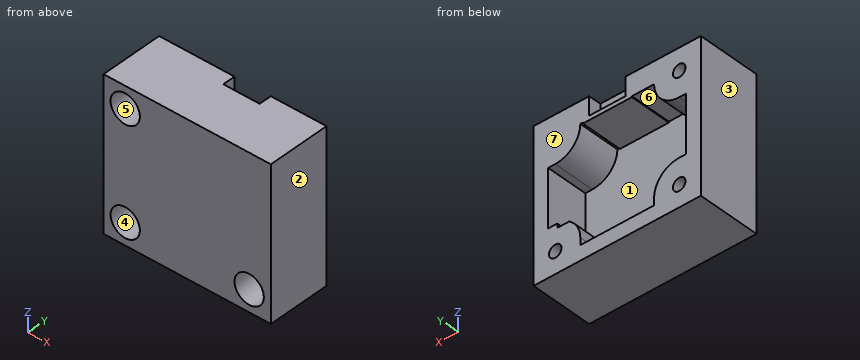
Autodesk Inventor part; units mm, degrees
ref_plane "YZ Plane" through (0, 0, 0) normal (1, 0, 0) x (0, 1, 0)
ref_plane "XZ Plane" through (0, 0, 0) normal (0, 1, 0) x (-1, 0, 0)
ref_plane "XY Plane" through (0, 0, 0) normal (0, 0, 1) x (1, 0, 0)
sketch "Эскиз1" plane through (0, 0, 0) normal (0, 1, 0) x (-1, 0, 0)
  line L0 (18, -16) -> (-18, -16)
  line L1 (-18, -16) -> (-18, 16)
  line L2 (-18, 16) -> (18, 16)
  line L3 (18, 16) -> (18, -16)
  line L4 (0, -25.2) -> (0, 25.2)
  line L5 (28, 0) -> (-28, 0)
  line L6 (14.82, -12.82) -> (-14.82, -12.82)
  line L7 (-14.82, -12.82) -> (-14.82, 12.82)
  line L8 (-14.82, 12.82) -> (14.82, 12.82)
  line L9 (14.82, 12.82) -> (14.82, -12.82)
  circle A0 centre (14.82, -12.82) radius 1.5
  circle A1 centre (14.82, 12.82) radius 1.5
  circle A2 centre (-14.82, 12.82) radius 1.5
  circle A3 centre (-14.82, -12.82) radius 1.5
  arc A4 (14.82, -6.82) -> (8.82, -12.82) centre (14.82, -12.82) ccw
  arc A5 (-8.82, -12.82) -> (-14.82, -6.82) centre (-14.82, -12.82) ccw
  arc A6 (8.82, 12.82) -> (14.82, 6.82) centre (14.82, 12.82) ccw
  arc A7 (-14.82, 6.82) -> (-8.82, 12.82) centre (-14.82, 12.82) ccw
  line L10 (20, -18) -> (-20, -18)
  line L11 (-20, -18) -> (-20, 18)
  line L12 (-20, 18) -> (20, 18)
  line L13 (20, 18) -> (20, -18)
  line L14 (-8.82, -12.82) -> (-8.82, -16)
  line L15 (8.82, -12.82) -> (8.82, -16)
  line L16 (14.82, -6.82) -> (18, -6.82)
  line L17 (14.82, 6.82) -> (18, 6.82)
  line L18 (8.82, 12.82) -> (8.82, 16)
  line L19 (-14.82, -6.82) -> (-20, -6.82)
  line L20 (-14.82, 6.82) -> (-20, 6.82)
  line L21 (-8.82, 12.82) -> (-8.82, 18)
  line L22 (-18, -6.82) -> (-18, 6.82)
  line L23 (8.82, 16) -> (-8.82, 16)
  line L24 (2, 13.6) -> (-6.7, 13.6)
  line L25 (-6.7, 13.6) -> (-6.7, 18)
  line L26 (3.5, 16) -> (3.5, 12.6)
  line L27 (3.5, 12.6) -> (-8.2, 12.6)
  line L28 (-8.2, 12.6) -> (-8.2, 16)
  line L29 (2, 13.6) -> (2, 18)
  circle A8 centre (-14.82, -12.82) radius 3.5
  circle A9 centre (14.82, -12.82) radius 3.5
  circle A10 centre (14.82, 12.82) radius 3.5
  circle A11 centre (-14.82, 12.82) radius 4
  line L30 (18, 6.82) -> (16.5, 6.82)
  line L31 (16.5, 6.82) -> (16.5, -6.82)
  line L32 (16.5, -6.82) -> (18, -6.82)
  line L33 (18, -6.82) -> (18, 6.82)
  line L34 (8.82, 16) -> (3.5, 16)
  line L35 (3.5, 16) -> (3.5, 14.5)
  line L36 (3.5, 14.5) -> (8.82, 14.5)
  line L37 (8.82, 14.5) -> (8.82, 16)
  line L38 (-8.2, 16) -> (-8.82, 16)
  line L39 (-8.82, 16) -> (-8.82, 14.5)
  line L40 (-8.82, 14.5) -> (-8.2, 14.5)
  line L41 (-8.2, 14.5) -> (-8.2, 16)
  line L42 (-18, 6.82) -> (-16.5, 6.82)
  line L43 (-16.5, 6.82) -> (-16.5, -6.82)
  line L44 (-16.5, -6.82) -> (-18, -6.82)
  line L45 (-18, -6.82) -> (-18, 6.82)
  line L46 (8.82, -16) -> (-8.82, -16)
  line L47 (-8.82, -16) -> (-8.82, -14.41)
  line L48 (8.82, -14.41) -> (8.82, -16)
  line L49 (8.82, -16) -> (-8.82, -16)
  line L50 (-8.82, -16) -> (-8.82, -14.5)
  line L51 (-8.82, -14.5) -> (8.82, -14.5)
  line L52 (8.82, -14.5) -> (8.82, -16)
  line L53 (-11.5034, -7.82) -> (-14.32, -7.82)
  line L54 (-14.32, -7.82) -> (-14.32, -6.8409)
  point P0 (0, 0)
  point P1 (-13.034, 10.913)
  dimension "d0" = 36
  dimension "d1" = 32
  dimension "d2" = 3.18
  dimension "d3" = 3.18
  dimension "d4" = 3.18
  dimension "d5" = 3.18
  dimension "d6" = 3
  dimension "d7" = 3
  dimension "d8" = 3
  dimension "d9" = 3
  dimension "d10" = 12
  dimension "d11" = 12
  dimension "d12" = 12
  dimension "d13" = 12
  dimension "d22" = 4.966
  dimension "d23" = 5.087
  dimension "d26" = 2
  dimension "d27" = 2
  dimension "d28" = 2
  dimension "d29" = 2
  dimension "d40" = 11.3
  dimension "d41" = 2.4
  dimension "d43" = 1
  dimension "d44" = 1.5
  dimension "d45" = 1.5
  dimension "d46" = 16
  dimension "d49" = 7
  dimension "d50" = 7
  dimension "d51" = 7
  dimension "d52" = 8
  dimension "d63" = 1.5
  dimension "d64" = 1.5
  dimension "d65" = 1.5
  dimension "d66" = 1.5
  dimension "d67" = 1.5
  dimension "d68" = 0.5
  dimension "d69" = 5
extrude "Выдавливание1" add sketch "Эскиз1" along normal blind 15 contours L3 A9 L5 L13 L10 L4 L0 | L0 A9 L3 | A9 L0 | L0 A9 L6 A0 L9 L3 | L3 A9 | L0 L15 L6 A9 | A9 L9 L16 L3 | L0 L4 L51 L15 | A9 L9 A0 L6 | L6 A4 L9 A9 | L16 L31 L5 L3 | L4 L10 L11 L19 L1 A8 L0 | L0 L14 L51 L4 | A0 L9 L6 | L6 L9 A0 | L5 L31 L17 L3 | L3 A10 L2 L29 L12 L13 L5 | L0 A8 L6 L14 | L17 L9 A10 L3 | A8 L0 | L0 A8 L1 L7 A3 L6 | L6 A8 L7 A5 L54 L53 | A10 L9 A1 L8 L2 L3 | L3 A10 | A6 L8 A10 L9 | L0 L1 A8 | L6 A3 L7 A8 | L11 L5 L1 L19 | L27 L28 L8 L4 | L4 L8 L26 L27 | L53 L54 A5 | A10 L2 L3 | A10 L8 A1 L9 | L29 L2 L4 L12 | L18 L2 A10 L8 | L8 L26 L36 L18 | A8 L1 | A3 L7 L6 | L6 L7 A3 | A8 L1 L19 L7 | L11 L20 L1 L5 | L1 L5 L43 L19 | L8 L28 L2 L25 L24 L4 | L4 L24 L29 L2 L26 L8 | L5 L1 L20 L43 | L20 L1 A11 L7 | L7 A11 L8 A7 | L2 A10 | A1 L8 L9 | L9 L8 A1 | L4 L2 L25 L12 | L29 L24 L4 L2 | L36 L26 L2 L18 | L11 L12 L21 L2 A11 L1 L20 | L24 L25 L2 L4 | L8 L21 L40 L28 | A11 L1 L2 L8 A2 L7 | L7 A2 L8 A11 | L8 A11 L2 L21 | L25 L2 L21 L12 | L40 L21 L2 L28 | A2 L8 L7 | L7 L8 A2 | A11 L1 | L1 L2 A11 | L2 A11
extrude "Выдавливание2" add sketch "Эскиз1" along normal blind 5
sketch "Эскиз2" plane through (0, 15, 0) normal (0, 1, 0) x (1, 0, 0)
  circle A0 centre (-14.82, -12.82) radius 1.5
  circle A1 centre (14.82, -12.82) radius 1.5
  circle A2 centre (14.82, 12.82) radius 1.5
  circle A3 centre (-14.82, 12.82) radius 1.5
  point P0 (0, 0)
extrude "Выдавливание3" cut sketch "Эскиз2" against normal up to next contours A0 | A2 | A3
extrude "Выдавливание5" cut sketch "Эскиз1" along normal blind 7 contours A9 L0 | L0 A9 L6 A0 L9 L3 | L3 A9 | A9 L9 A0 L6 | A8 L0 | L0 A8 L1 L7 A3 L6 | A10 L9 A1 L8 L2 L3 | L3 A10 | L6 A3 L7 A8 | A10 L8 A1 L9 | A8 L1 | L2 A10
sketch "Эскиз3" plane through (0, 15, 0) normal (0, 1, 0) x (1, 0, 0)
  line L0 (-20, -18) -> (20, -18)
  line L1 (-2, -13.6) -> (-2, -18)
  line L2 (-2, -13.6) -> (6.7, -13.6)
  line L3 (6.7, -13.6) -> (6.7, -18)
  point P0 (0, 0)
extrude "Выдавливание6" cut sketch "Эскиз3" against normal blind 3
sketch "Эскиз4" plane through (0, 15, 0) normal (0, 1, 0) x (1, 0, 0)
  line L0 (11.5034, 7.82) -> (14.32, 7.82)
  line L1 (14.32, 7.82) -> (14.32, 6.8409)
  arc A0 (8.82, 12.82) -> (14.82, 6.82) centre (14.82, 12.82) ccw
  point P0 (0, 0)
extrude "Выдавливание7" cut sketch "Эскиз4" against normal up to surface (10 mm away)
properties part number "case_top" material "Polycarbonate, Clear"
Design review of the part built by this model. Coordinates are the model's own, in mm. Face numbers are marked on the shaded views. A direction names the side the tool comes from. Round coordinates to 2 decimals unless told otherwise and drop trailing zeros. Write each loop counter-clockwise with the first axis right and the second up, starting at its lowest first coordinate (ties: lowest second). Pieces come first, ordered by that corner, then holes. Notation, with made-up numbers: (40.5, 39.5) - (46.5, 39.5) arc R22 ccw to (46.5, 48.5) - close; hole circle Ø7 at (64.5, 16.25). An arc over 180 degrees is marked (long way). Use a Markdown table: item, result. Add a question column.
1. We need section C-C (x = 4). State the section outline as (y, z) points.
2. We need section A-A (y = 3.75). State the section outline as (x, z) points, then the cut area to 3 significant figures.
3. We need section B-B (z = 1). State the section outline as (x, y) points.
4. Mouldability with a two-part tool opening along X and no side actions: class the marked faces 1, 2, 3 and 4 as +X half, -X half, draft (parallel to the pull), parting line (faces both ways), or undercut.
5. Clearance check with flat-ended pins moving along their axes: pin 1 (13.5 mm diameter, centred on x = 1, z = -2, fed in from +Y); pin 2 (7.5 mm diameter, centred on x = -13, z = -12.5, fed in from -Y); pin 3 (3.5 mm diameter, centred on x = -14.82, z = 12.82, fed in from -Y); pin 4 (1.5 mm diameter, centred on x = 2.5, y = 13.5, fed in from +Z). State where each tip first meets the part, or that it passes through.
6. We need section D-D (y = 10.75). State the section outline as (x, z) points.
7. For the marked faces 5, 6 and 7, list the 3-axis set-ups (+Z, -Z, +X, -X, +Y, -Y) from which the entire face can be reached by the end or side of a thin tool; tool diameter is ignored.
8. Wall thickness on probe 1 along Z at (x, y) = (-14.82, 5.5); probe 2 along Z at (x, y) = (-14.82, 4); probe 3 along Z at (x, y) = (14.82, 9.25): over which ranges is each line inside the solid? List them lowest first.
Output:
| question | item | result |
|---|---|---|
| 1 | outline | (0, -18) - (15, -18) - (15, -14.5) - (5, -14.5) - (5, 12.6) - (15, 12.6) - (15, 13.6) - (12, 13.6) - (12, 18) - (0, 18) - close |
| 2 | outline | (-20, -18) - (20, -18) - (20, 18) - (-20, 18) - close; hole circle Ø7 at (-14.82, -12.82); hole circle Ø7 at (-14.82, 12.82); hole circle Ø7 at (14.82, -12.82) |
| 2 | area | 1,320 mm2 |
| 3 | outline | (-20, 0) - (20, 0) - (20, 15) - (16.5, 15) - (16.5, 5) - (-16.5, 5) - (-16.5, 15) - (-20, 15) - close |
| 4 | face 1 | undercut |
| 4 | face 2 | +X half |
| 4 | face 3 | -X half |
| 4 | face 4 | undercut |
| 5 | pin 1 | stops at y = 5 |
| 5 | pin 2 | stops at y = 0 |
| 5 | pin 3 | stops at y = 7 |
| 5 | pin 4 | stops at z = 13.6 |
| 6 | outline | (-20, -18) - (20, -18) - (20, 18) - (-20, 18) - close; hole (-16.5, -6.82) - (-14.82, -6.82) arc R6 cw to (-8.82, -12.82) - (-8.82, -14.5) - (8.82, -14.5) - (8.82, -12.82) arc R6 cw to (11.5, -7.82) - (14.32, -7.82) - (14.32, -6.84) arc R6 cw to (14.82, -6.82) - (16.5, -6.82) - (16.5, 6.82) - (14.82, 6.82) arc R6 cw to (8.82, 12.82) - (8.2, 12.82) - (8.2, 12.6) - (-3.5, 12.6) - (-3.5, 12.82) - (-8.82, 12.82) arc R6 cw to (-14.82, 6.82) - (-16.5, 6.82) - close; hole circle Ø3 at (-14.82, -12.82); hole circle Ø3 at (-14.82, 12.82); hole circle Ø3 at (14.82, -12.82) |
| 7 | face 5 | -Y |
| 7 | face 6 | +Y |
| 7 | face 7 | +Z, -Z, +X, -X, +Y |
| 8 | probe 1 | z = -18 to -16.32, -9.32 to -6.82, 6.82 to 9.32, 16.32 to 18 |
| 8 | probe 2 | z = -18 to -16.32, -9.32 to 9.32, 16.32 to 18 |
| 8 | probe 3 | z = -18 to -14.32, -11.32 to -6.82, 6.82 to 18 |
